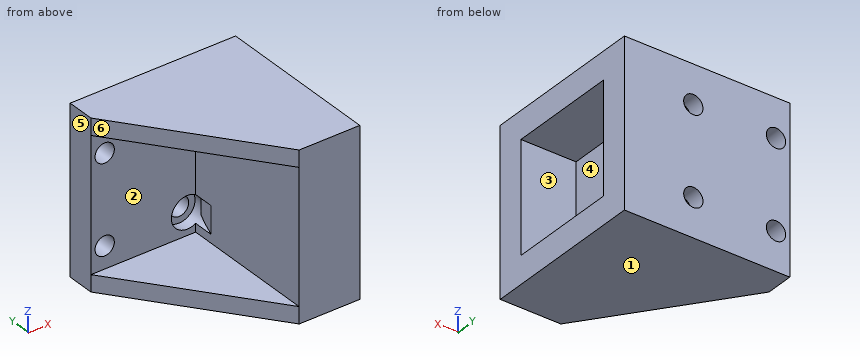
```python
from build123d import *

# Parameters (mm, degrees)
SKETCH1_W           = 30
SKETCH1_H           = 30
SKETCH1_R           = 1.75
BOSS_EXTRUDE1_DEPTH = 5
SKETCH2_W           = 11
SKETCH2_H           = 30
BOSS_EXTRUDE2_DEPTH = 25
SKETCH3_W           = 20
SKETCH3_H           = 20
CUT_EXTRUDE1_DEPTH  = 10
BOSS_EXTRUDE3_DEPTH = 3
BOSS_EXTRUDE4_DEPTH = 3
SKETCH12_R          = 2.9
CUT_EXTRUDE3_DEPTH  = 2
CHAMFER3_SIZE       = 3.732050808
CHAMFER3_SIZE_2     = 1


with BuildPart() as part:
    # Sketch1 → Boss-Extrude1 (new body)
    with BuildSketch(Plane(origin=(0, 0, 0), x_dir=(1, 0, 0), z_dir=(0, 1, 0))):
        with Locations((15, 15)):
            Rectangle(SKETCH1_W, SKETCH1_H)
        with Locations(Location((2.5, 7, 0), (0, 0, 270))):
            Circle(SKETCH1_R, mode=Mode.SUBTRACT)
        with Locations(Location((17.5, 7, 0), (0, 0, 270))):
            Circle(SKETCH1_R, mode=Mode.SUBTRACT)
        with Locations(Location((2.5, 23, 0), (0, 0, 270))):
            Circle(SKETCH1_R, mode=Mode.SUBTRACT)
        with Locations(Location((17.5, 23, 0), (0, 0, 270))):
            Circle(SKETCH1_R, mode=Mode.SUBTRACT)
    extrude(amount=BOSS_EXTRUDE1_DEPTH)

    # Sketch2 → Boss-Extrude2 (add)
    with BuildSketch(Plane.XZ):
        with Locations((24.5, -15)):
            Rectangle(SKETCH2_W, SKETCH2_H)
    extrude(amount=BOSS_EXTRUDE2_DEPTH)

    # Sketch3 → Cut-Extrude1 (cut)
    with BuildSketch(Plane(origin=(30, 0, 0), x_dir=(0, 0, -1), z_dir=(1, 0, 0))):
        with Locations((15, -10)):
            Rectangle(SKETCH3_W, SKETCH3_H)
    extrude(amount=-CUT_EXTRUDE1_DEPTH, mode=Mode.SUBTRACT)

    # Sketch8 → Boss-Extrude3 (add)
    with BuildSketch(Plane(origin=(0, 0, -30), x_dir=(-1, 0, 0), z_dir=(0, 0, -1))):
        Polygon((-19, 0), (0, 0), (-19, -25), align=None)
    extrude(amount=-BOSS_EXTRUDE3_DEPTH)

    # Sketch11 → Boss-Extrude4 (add)
    with BuildSketch(Plane.XY):
        Polygon((19, -25), (0, 0), (19, 0), align=None)
    extrude(amount=-BOSS_EXTRUDE4_DEPTH)

    # Sketch12 → Cut-Extrude3 (cut)
    with BuildSketch(Plane.XZ):
        with Locations(Location((17.5, -23, 0), (0, 0, 270))):
            Circle(SKETCH12_R)
        with Locations(Location((17.5, -7, 0), (0, 0, 270))):
            Circle(SKETCH12_R)
    extrude(amount=-CUT_EXTRUDE3_DEPTH, mode=Mode.SUBTRACT)

    # Chamfer3
    # the kernel refuses this chamfer: 3.732050808, 1 mm, written as the material it takes off along each edge
    with BuildSketch(Plane(origin=(19, 0, -10.826968438), x_dir=(-0.009967146577155864, -0.9999503267608394, 0), z_dir=(0, 0, -1))) as chamfer3_piece_1_section:
        Polygon((CHAMFER3_SIZE * 0.999950326645, -CHAMFER3_SIZE * 0.009967146576), (-CHAMFER3_SIZE_2 * 0.00996714657716, -CHAMFER3_SIZE_2 * 0.999950326761), (0, 0), align=None)
    chamfer3_piece_1 = extrude(amount=24.346063125, mode=Mode.PRIVATE)
    chamfer3_piece_1 = chamfer3_piece_1 & Plane(origin=(17.5, -1.271193321, -23), x_dir=(0, 0, -1), z_dir=(0, -1, 0)) * Cylinder(2.9, 64, mode=Mode.PRIVATE)
    add(chamfer3_piece_1, mode=Mode.SUBTRACT)
    with BuildSketch(Plane(origin=(19, 0, 5.173031562), x_dir=(-0.009967146577155864, -0.9999503267608394, 0), z_dir=(0, 0, -1))) as chamfer3_piece_2_section:
        Polygon((CHAMFER3_SIZE * 0.999950326645, -CHAMFER3_SIZE * 0.009967146576), (-CHAMFER3_SIZE_2 * 0.00996714657716, -CHAMFER3_SIZE_2 * 0.999950326761), (0, 0), align=None)
    chamfer3_piece_2 = extrude(amount=24.346063125, mode=Mode.PRIVATE)
    chamfer3_piece_2 = chamfer3_piece_2 & Plane(origin=(17.5, -1.525075197, -7), x_dir=(0, 0, -1), z_dir=(0, -1, 0)) * Cylinder(2.9, 64, mode=Mode.PRIVATE)
    add(chamfer3_piece_2, mode=Mode.SUBTRACT)


solid = part.part
```
Build history of the part. All positions in model axes, mm. Face numbers are marked on the shaded views. A direction names the side the tool comes from. Round coordinates to 2 decimals unless told otherwise and drop trailing zeros. Loops run counter-clockwise (first coordinate to the right, second up) from the corner with the lowest first, then second, coordinate; pieces in that order, holes last.
Item 1: Drill centre lines: line 1 along Z through (x, y) = (17.5, 2.8); line 2 along X through (y, z) = (3.9, -7); line 3 along X through (y, z) = (1.85, -23). Where is each one in solid material? Low to high.
Item 2: Saw through at A-A (y = 1). List the corners of the cut face in (x, z), then the cut area to 3 significant figures.
Item 3: Saw through at B-B (z = -23). List the corners of the cut face in (x, y).
Item 4: Saw through at C-C (y = -4.75). List the corners of the cut face in (x, z), then the cut area to 3 significant figures.
Item 5: Pin check, flat tips, straight feed: P1, Ø9.5, axis at x = 17.5, z = -23, coming from the +Y side; P2, Ø8, axis at x = 5, y = -18, coming from the -Z side; P3, Ø1, axis at x = 6.5, z = -5.5, coming from the -Y side; P4, Ø1.7, axis at x = 16, z = -6.5, coming from the -Y side. Stop position of each tip, or through.
Item 6: Two-plate mould, pull along Y, no slides. Class the marked faces 4, 5 and 6: released by +Y, released by -Y, zero draft, split by the parting line, or undercut.
Item 7: Which spindle directions (+Z, -Z, +X, -X, +Y, -Y) get a long thin tool onto all of the face, cutting with end or side? Do the marked faces 1, 2 and 3. Say none if no direction does.
Item 8: Saw through at D-D (z = -18). List the corners of the cut face in (x, y).
Worked answers:
1. line 1: z = -30 to -24.75, -21.25 to -8.75, -5.25 to 0
1. line 2: x = 0 to 0.75, 4.25 to 15.75, 19.25 to 30
1. line 3: x = 0 to 0.75, 4.25 to 14.6, 20.4 to 30
2. outline: (0, -30) - (30, -30) - (30, 0) - (0, 0) - close; hole circle Ø3.5 at (2.5, -23); hole circle Ø3.5 at (2.5, -7); hole circle Ø5.8 at (17.5, -23); hole circle Ø5.8 at (17.5, -7)
2. area: 828 mm2
3. outline: (0, 0) - (0.75, 0) - (0.75, 5) - (0, 5) - close; (4.25, 0) - (14.6, 0) - (14.6, 2) - (15.75, 2) - (15.75, 5) - (4.25, 5) - close; (19, -25) - (30, -25) - (30, -20) - (20, -20) - (20, 0) - (19, -3.73) - close; (19.25, 2) - (20.4, 2) - (20.4, 0) - (30, 0) - (30, 5) - (19.25, 5) - close
4. outline: (3.61, -30) - (30, -30) - (30, -25) - (20, -25) - (20, -5) - (30, -5) - (30, 0) - (3.61, 0) - (3.61, -3) - (19, -3) - (19, -27) - (3.61, -27) - close
4. area: 222 mm2
5. P1: stops at y = 5
5. P2: passes through
5. P3: stops at y = 0
5. P4: stops at y = 2
6. face 4: undercut
6. face 5: zero draft
6. face 6: released by -Y
7. face 1: -Z, +X, -X, +Y, -Y
7. face 2: -X, -Y
7. face 3: +X
8. outline: (0, 0) - (19, 0) - (19, -25) - (30, -25) - (30, -20) - (20, -20) - (20, 0) - (30, 0) - (30, 5) - (0, 5) - close
